Autodesk Inventor part; units mm, degrees
ref_plane "YZ Plane" through (0, 0, 0) normal (1, 0, 0) x (0, 1, 0)
ref_plane "XZ Plane" through (0, 0, 0) normal (0, 1, 0) x (-1, 0, 0)
ref_plane "XY Plane" through (0, 0, 0) normal (0, 0, 1) x (1, 0, 0)
sketch "Sketch1" plane through (0, 0, 0) normal (0, 1, 0) x (-1, 0, 0)
  line L0 (0, 0) -> (25, 0)
  line L1 (25, 0) -> (25, -81)
  line L2 (25, -81) -> (0, -81)
  line L3 (0, -81) -> (0, 0)
  dimension "d0" = 25
  dimension "d1" = 81
extrude "Extrusion1" add sketch "Sketch1" along normal blind 25
sketch "Sketch2" plane through (0, 0, 0) normal (1, 0, 0) x (0, 0, -1)
  line L0 (81, 0) -> (81, 10)
  line L1 (81, 0) -> (81, 25)
  line L2 (81, 25) -> (21, 25)
  line L3 (21, 25) -> (21, 10)
  line L4 (21, 10) -> (81, 10)
  line L5 (81, 10) -> (81, 25)
  point P0 (0, 0)
  dimension "d4" = 10
  dimension "d5" = 60
extrude "Extrusion2" cut sketch "Sketch2" against normal through all
sketch "Sketch3" plane through (0, 10, -21) normal (0, 1, 0) x (1, 0, 0)
  line L0 (0, 60) -> (0, -21)
  line L1 (-25, 60) -> (0, 60)
  line L2 (0, 60) -> (0, 35)
  line L3 (0, 35) -> (-25, 35)
  line L4 (-25, 35) -> (-25, 60)
  circle A0 centre (-12.5, 47.5) radius 11.125
  dimension "d8" = 25
  dimension "d9" = 22.25
extrude "Extrusion3" cut sketch "Sketch3" against normal blind 7 contours A0
sketch "Sketch4" plane through (-25, 0, 0) normal (0, 0, 1) x (1, 0, 0)
  line L0 (25, 10) -> (0, 25)
  line L1 (0, 25) -> (25, 25)
  line L2 (0, 25) -> (25, 25)
  line L3 (25, 25) -> (25, 10)
  point P0 (25, 0)
extrude "Extrusion4" cut sketch "Sketch4" against normal blind 21
sketch "Sketch5" plane through (0, 0, 0) normal (0, -1, 0) x (1, 0, 0)
  line L0 (0, 0) -> (-25, 0)
  line L1 (-10.5, -162) -> (-14.5, -162)
  line L2 (-14.5, -162) -> (-14.5, 0)
  line L3 (-14.5, 0) -> (-10.5, 0)
  line L4 (-10.5, 0) -> (-10.5, -162)
  line L5 (-25, -81) -> (0, -81)
  line L6 (-10.5, -162) -> (-14.5, 0) construction
  line L7 (-14.5, -162) -> (-10.5, 0) construction
  point P0 (-12.5, -81)
  dimension "d14" = 4
extrude "Extrusion5" cut sketch "Sketch5" against normal blind 2
sketch "Sketch6" plane through (-25, 10, -81) normal (0, 1, 0) x (1, 0, 0)
  line L0 (25, -25) -> (0, -25)
  line L1 (0, -25) -> (0, 0)
  line L2 (0, 0) -> (25, 0)
  line L3 (25, 0) -> (25, -25)
  circle A0 centre (12.5, -12.5) radius 11.125
  line L4 (25, -25) -> (0, 0) construction
  line L5 (0, -25) -> (25, 0) construction
  circle A1 centre (12.5, -12.5) radius 11.125
  point P0 (25, -81)
extrude "Extrusion6" add sketch "Sketch6" along normal blind 2
sketch "Sketch7" plane through (-12.5, 3, -68.5) normal (0, 1, 0) x (1, 0, 0)
  circle A0 centre (0, 0) radius 11.125
  circle A1 centre (0, 0) radius 11.125
  point P0 (12.5, -68.5)
extrude "Extrusion7" add sketch "Sketch7" along normal blind 2
sketch "Sketch8" plane through (-25, 0, 0) normal (0, 0, 1) x (1, 0, 0)
  line L0 (0, 0) -> (0, 50)
  line L1 (0, 50) -> (25, 50)
  line L2 (25, 50) -> (25, 37)
  line L3 (25, 37) -> (0, 50)
  line L4 (25, 37) -> (25, 10)
  line L5 (25, 0) -> (25, 12)
  line L6 (25, 10) -> (0, 25)
  line L7 (25, 10) -> (0, 25)
  line L8 (0, 50) -> (0, 25)
  line L9 (25, 10) -> (0, 25)
  line L10 (25, 37) -> (25, 10)
  line L11 (25, 10) -> (0, 10)
  line L12 (25, 37) -> (0, 50)
  dimension "d21" = 50
  dimension "d22" = 13
extrude "Extrusion8" add sketch "Sketch8" against normal blind 15 contours L0 L3 L4 L6
sketch "Sketch9" plane through (-25, 0, -81) normal (-1, 0, 0) x (0, 0, 1)
  line L0 (66, 25) -> (60, 25)
  line L1 (60, 25) -> (60, 10)
  line L2 (60, 10) -> (66, 10)
  line L3 (66, 10) -> (66, 25)
  point P0 (81, 0)
extrude "Extrusion9" cut sketch "Sketch9" against normal through all
sketch "Sketch10" plane through (-25, 0, -15) normal (0, 0, -1) x (-1, 0, 0)
  point P0 (-25, 0)
sketch "Sketch11" plane through (-10.5, 0, 0) normal (0, 0, 1) x (1, 0, 0)
  line L0 (10.5, 10) -> (-2, 10)
  line L1 (-2, 10) -> (-2, 47.9639)
  line L2 (-2, 47.9639) -> (10.5, 47.9639)
  line L3 (10.5, 47.9639) -> (10.5, 10)
  point P0 (10.5, 0)
extrude "Extrusion10" cut sketch "Sketch11" against normal blind 15
sketch "Sketch12" plane through (0, 0, 0) normal (0, 0, 1) x (1, 0, 0)
  line L0 (-12.5, 43.5) -> (-37.3421, 56.4179)
  line L1 (-25, 50) -> (-12.5, 43.5)
  line L2 (-37.3421, 56.4179) -> (-37.3421, 50)
  line L3 (-37.3421, 50) -> (-25, 40.4241)
  line L4 (-25, 0) -> (-25, 50)
  line L5 (-12.5, 43.5) -> (-25, 40.4241)
  point P0 (0, 0)
  dimension "d29" = 28
extrude "Extrusion11" add sketch "Sketch12" against normal blind 15 contours L4 L3 L2 L0
fillet "Fillet1" radius 2 1 edges at (-24.921, 49.9589, 0)
fillet "Fillet2" radius 2 1 edges at (-31.171, 45.212, 0)
fillet "Fillet3" radius 2 2 edges at (-24.921, 49.9589, -15) (-31.171, 45.212, -15)
sketch "Sketch13" plane through (0, 0, 0) normal (0, 0, 1) x (1, 0, 0)
  line L0 (-10.5, 2) -> (-16.5509, 12)
  line L1 (-23.625, 12) -> (-1.375, 12)
  line L2 (-16.5509, 12) -> (-16.5509, 42.153)
  line L3 (-16.5509, 42.153) -> (-20.5509, 42.153)
  line L4 (-20.5509, 42.153) -> (-20.5509, 12)
  line L5 (-20.5509, 12) -> (-14.5, 2)
  line L6 (-14.5, 2) -> (-10.5, 2)
  line L7 (-14.5, 2) -> (-10.5, 2)
  point P0 (0, 0)
  dimension "d35" = 4
extrude "Extrusion12" cut sketch "Sketch13" against normal blind 2
fillet "Fillet4" radius 2 1 edges at (-18.5509, 42.153, 0)
sketch "Sketch14" plane through (0, 10, 0) normal (0, 1, 0) x (1, 0, 0)
  line L0 (0, 56) -> (-25, 56)
  line L1 (0, 0) -> (-4, 0)
  line L2 (-4, 0) -> (-4, 56)
  line L3 (-4, 56) -> (0, 56)
  line L4 (0, 56) -> (0, 0)
  dimension "d39" = 4
extrude "Extrusion13" cut sketch "Sketch14" against normal through all
sketch "Sketch15" plane through (-25, 0, -15) normal (0, 0, -1) x (-1, 0, 0)
  point P0 (-25, 0)
properties part number "ConductiveThread"
Work out the finished part from the listing and answer in its coordinate system (mm). A direction names the side the tool comes from. Coordinates: 2 decimals unless noted, no trailing zeros. Loops run counter-clockwise (first coordinate to the right, second up) from the corner with the lowest first, then second, coordinate; pieces in that order, holes last. Notation, with made-up numbers: (5.25, -34) -> (14.25, -34) arc R15 ccw to (14.25, -25) -> close; hole circle Ø6 at (62, 16). An arc over 180 degrees is marked (long way). Answer as CSV lines item,"result".
Q1. Find the intervals of material crossed by probe 1 along X at (y, z) = (9, -68.5) (3 decimals); probe 2 along Z at (x, y) = (-12.5, 7.5) (3 decimals); probe 3 along Z at (x, y) = (-24.5, 16.5), in increasing order.
Findings:
probe 1,"x = -25 to -23.625, -1.375 to 0"
probe 2,"z = -81 to -79.625, -57.375 to 0"
probe 3,"z = -15 to 0"
Q2. The part is cut by section C-C on y = 29.5. Write down the section's boundary in (x, z), and give its area (4 significant figures).
Findings:
outline,"(-25, -15) -> (-12.5, -15) -> (-12.5, 0) -> (-16.55, 0) -> (-16.55, -2) -> (-20.55, -2) -> (-20.55, 0) -> (-25, 0) -> close"
area,"179.5 mm²"
Q3. The part is cut by section D-D on x = -6.5. Write down the section's boundary in (y, z), and give its area (3 significant figures).
Findings:
outline,"(0, -81) -> (12, -81) -> (12, -77.87) -> (5, -77.87) -> (5, -59.13) -> (12, -59.13) -> (12, -56) -> (10, -56) -> (10, 0) -> (0, 0) -> close"
area,"729 mm²"
Q4. Each of these flat-tipped pins is pushed along its axis until it touches: pin 1 (2 mm diameter, centred on y = 36, z = -1.5, fed in from +X); pin 2 (1.5 mm diameter, centred on y = 12.5, z = -55, fed in from -X); pin 3 (4 mm diameter, centred on y = 43, z = -15, fed in from -X); pin 4 (4 mm diameter, centred on y = 7.5, z = -24.5, fed in from +X). Where does it stop, or does it pass through?
Findings:
pin 1,"stops at x = -12.5"
pin 2,"passes through"
pin 3,"stops at x = -30.12"
pin 4,"stops at x = -4"
Q5. For a pull along Z with two mould halves and no side action, classify faces 1 (the face through (-6, 0, -40)), 2 (the face through (-18.523, 42.754, -0.57)), 3 (the face through (-13, 6, -81)), 4 (the face through (-15, 10, -28)) as +Z half, -Z half, draft (parallel to the pull), parting line (faces both ways), or undercut.
Findings:
face 1,"draft"
face 2,"+Z half"
face 3,"-Z half"
face 4,"undercut"
Q6. A tool of negligible diameter and unlimited length cuts with its end or side. For faces 5 (the face through (-13.95, 8.45, -57.47)), 6 (the face through (-4, 5, -28)), 7 (the face through (-10.5, 1, -40)), 8 (the face through (-17.57, 7.07, -0.99)), from which of +Z, -Z, +X, -X, +Y, -Y can it reach the whole face along a straight path? Write none if from no direction.
Findings:
face 5,"+Y"
face 6,"+Z, +X, +Y, -Y"
face 7,"+Z, -Z, -Y"
face 8,"+Z"
Q7. The part is cut by section B-B on y = 11. Write down the section's boundary in (x, z) (3 decimals).
Findings:
outline,"(-25, -81) -> (0, -81) -> (0, -56) -> (-25, -56) -> close; (-25, -15) -> (-12.5, -15) -> (-12.5, 0) -> (-15.946, 0) -> (-15.946, -2) -> (-19.946, -2) -> (-19.946, 0) -> (-25, 0) -> close; hole circle Ø22.25 at (-12.5, -68.5)"
Q8. The part is cut by section A-A on z = -68.5. Write down the section's boundary in (x, y) (3 decimals), and give its area (3 significant figures).
Findings:
outline,"(-25, 0) -> (-14.5, 0) -> (-14.5, 2) -> (-10.5, 2) -> (-10.5, 0) -> (0, 0) -> (0, 12) -> (-1.375, 12) -> (-1.375, 5) -> (-23.625, 5) -> (-23.625, 12) -> (-25, 12) -> close"
area,"136 mm²"
